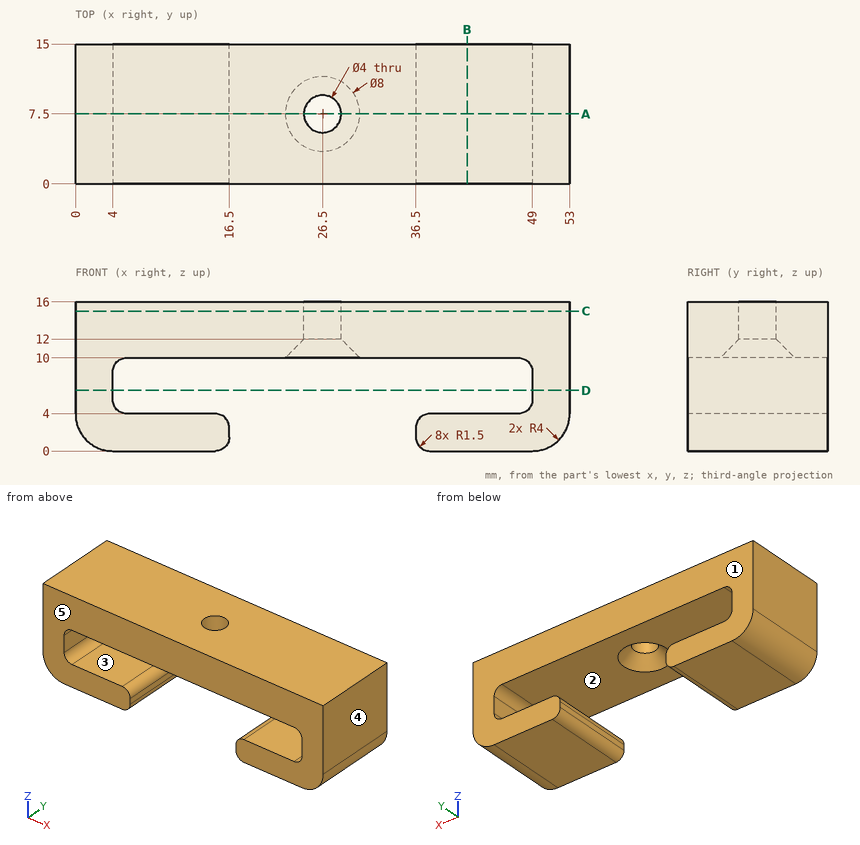
Part print with two shaded views. Sizes in mm from the minimum x, y, z corner. A direction names the side the tool comes from. Coordinates: 2 decimals unless noted, no trailing zeros. Write each loop counter-clockwise with the first axis right and the second up, starting at its lowest first coordinate (ties: lowest second). Pieces come first, ordered by that corner, then holes. Notation, with made-up numbers: (-11.5, 44.25) -> (32.5, 44.25) arc R9 ccw to (32.5, 58.25) -> close; hole circle Ø9 at (87.5, -34.5). An arc over 180 degrees is marked (long way). Return JSON: item names as keys, results as strings. Group by question number.
Q1. Which spindle directions (+Z, -Z, +X, -X, +Y, -Y) get a long thin tool onto all of the face, cutting with end or side? Do the marked faces 1 and 2. Say none if no direction does.
Q2. Drill centre lines: line 1 (X direction, y = 7.5, z = 15.05); line 2 (Z direction, x = 6.5, y = 1.75); line 3 (Y direction, x = 26.5, z = 13.2). Where is each one in solid material? Low to high.
Q3. Pull direction X, two halves, no side cores. Call the marked faces 3, 4 and 5: released by +X, released by -X, zero draft, split by the parting line, or undercut.
Q4. Cut at B-B, the plane x = 42. Give the cut face in (y, z), then the cut area to 3 significant figures.
Q5. Cut at C-C, the plane z = 15. Give the cut face in (x, y).
Q6. Flat gauge pins, fed straight in: pin 1 (8 mm diameter, centred on y = 5.5, z = 4.5, fed in from -X); pin 2 (7.5 mm diameter, centred on x = 26.5, y = 7, fed in from -Z); pin 3 (1.1 mm diameter, centred on y = 9.5, z = 2, fed in from -X). Where does each tip first touch, or does it go through?
Q7. Cut at A-A, the plane y = 7.5. Give the cut face in (x, z).
Q8. Cut at D-D, the plane z = 6.5. Give the cut face in (x, y), then the cut area to 3 significant figures.
Returned:
{
 "1": {"face 1": "+Z, -Z, +X, -X, +Y", "face 2": "+Y, -Y"},
 "2": {"line 1": "x = 0 to 24.5, 28.5 to 53", "line 2": "z = 0 to 4, 10 to 16", "line 3": "y = 0 to 5.5, 9.5 to 15"},
 "3": {"face 3": "undercut", "face 4": "released by +X", "face 5": "zero draft"},
 "4": {"outline": "(0, 0) -> (15, 0) -> (15, 4) -> (0, 4) -> close; (0, 10) -> (15, 10) -> (15, 16) -> (0, 16) -> close", "area": "150 mm2"},
 "5": {"outline": "(0, 0) -> (53, 0) -> (53, 15) -> (0, 15) -> close; hole circle Ø4 at (26.5, 7.5)"},
 "6": {"pin 1": "stops at x = 0", "pin 2": "stops at z = 10", "pin 3": "stops at x = 0.27"},
 "7": {"outline": "(0, 4) arc R4 ccw to (4, 0) -> (15, 0) arc R1.5 ccw to (16.5, 1.5) -> (16.5, 2.5) arc R1.5 ccw to (15, 4) -> (5.5, 4) arc R1.5 cw to (4, 5.5) -> (4, 8.5) arc R1.5 cw to (5.5, 10) -> (22.5, 10) -> (24.5, 12) -> (24.5, 16) -> (0, 16) -> close; (28.5, 12) -> (30.5, 10) -> (47.5, 10) arc R1.5 cw to (49, 8.5) -> (49, 5.5) arc R1.5 cw to (47.5, 4) -> (38, 4) arc R1.5 ccw to (36.5, 2.5) -> (36.5, 1.5) arc R1.5 ccw to (38, 0) -> (49, 0) arc R4 ccw to (53, 4) -> (53, 16) -> (28.5, 16) -> close"},
 "8": {"outline": "(0, 0) -> (4, 0) -> (4, 15) -> (0, 15) -> close; (49, 0) -> (53, 0) -> (53, 15) -> (49, 15) -> close", "area": "120 mm2"}
}
